```python
from build123d import *

# Parameters (mm, degrees)
SKETCH1_W                      = 60
SKETCH1_H                      = 397.5
BASE_FLANGE1_DEPTH             = 4
EDGE_FLANGE1_STRIP_W           = 18
EDGE_FLANGE1_STRIP_H           = 4
EDGE_FLANGE1_STRIP_CUT_DEPTH   = 397.5
EDGE_FLANGE1_DEPTH             = 397.5
EDGE_FLANGE2_STRIP_W           = 18
EDGE_FLANGE2_STRIP_H           = 4
EDGE_FLANGE2_STRIP_CUT_DEPTH   = 55
EDGE_FLANGE2_STRIP_2_W         = 18
EDGE_FLANGE2_STRIP_2_H         = 4
EDGE_FLANGE2_STRIP_CUT_2_DEPTH = 55
EDGE_FLANGE2_STRIP_3_W         = 18
EDGE_FLANGE2_STRIP_3_H         = 4
EDGE_FLANGE2_STRIP_CUT_3_DEPTH = 55
EDGE_FLANGE2_STRIP_4_W         = 18
EDGE_FLANGE2_STRIP_4_H         = 4
EDGE_FLANGE2_STRIP_CUT_4_DEPTH = 55
EDGE_FLANGE2_DEPTH             = 55
EDGE_FLANGE2_BEND_DEPTH        = 55
EDGE_FLANGE2_BEND_2_DEPTH      = 55
EDGE_FLANGE2_BEND_3_DEPTH      = 55
SKETCH18_R                     = 4.6
EXTRUDE1_DEPTH                 = 408.38464625
SKETCH19_R                     = 4.6
EXTRUDE2_DEPTH                 = 4
SKETCH20_R                     = 4.6
EXTRUDE3_DEPTH                 = 4


# Sheet-metal steps are written as plain solids
with BuildPart() as part:
    # Sketch1 → Base-Flange1 (new body)
    with BuildSketch(Plane(origin=(0, 0, 0), x_dir=(1, 0, 0), z_dir=(0, 1, 0))):
        Rectangle(SKETCH1_W, SKETCH1_H)
    extrude(amount=BASE_FLANGE1_DEPTH)

    # Edge-Flange1 strip (across the edge) → Edge-Flange1 strip cut (cut)
    with BuildSketch(Plane(origin=(-30, 4, -198.75), x_dir=(1, 0, 0), z_dir=(0, 0, 1))):
        with Locations((-4, -2)):
            Rectangle(EDGE_FLANGE1_STRIP_W, EDGE_FLANGE1_STRIP_H)
    extrude(amount=EDGE_FLANGE1_STRIP_CUT_DEPTH, mode=Mode.SUBTRACT)

    # Edge-Flange1 section (across the edge) → Edge-Flange1 (add)
    with BuildSketch(Plane(origin=(-30, 4, -198.75), x_dir=(1, 0, 0), z_dir=(0, 0, 1))):
        with BuildLine():
            Line((0, 1), (0, 56))
            Line((0, 56), (4, 56))
            Line((4, 56), (4, 1))
            ThreePointArc((4, 1), (4.292893219, 0.292893219), (5, 0))
            Line((5, 0), (5, -4))
            ThreePointArc((5, -4), (1.464466094, -2.535533906), (0, 1))
        make_face()
    extrude(amount=EDGE_FLANGE1_DEPTH)

    # Edge-Flange2 strip (across the edge) → Edge-Flange2 strip cut (cut)
    with BuildSketch(Plane(origin=(-30, 5, 198.75), x_dir=(0, 0, -1), z_dir=(0, 1, 0))):
        with Locations((-4, -2)):
            Rectangle(EDGE_FLANGE2_STRIP_W, EDGE_FLANGE2_STRIP_H)
    extrude(amount=EDGE_FLANGE2_STRIP_CUT_DEPTH, mode=Mode.SUBTRACT)

    # Edge-Flange2 strip 2 (across the edge) → Edge-Flange2 strip cut 2 (cut)
    with BuildSketch(Plane(origin=(30, 0, 198.75), x_dir=(0, 0, -1), z_dir=(-1, 0, 0))):
        with Locations((-4, -2)):
            Rectangle(EDGE_FLANGE2_STRIP_2_W, EDGE_FLANGE2_STRIP_2_H)
    extrude(amount=EDGE_FLANGE2_STRIP_CUT_2_DEPTH, mode=Mode.SUBTRACT)

    # Edge-Flange2 strip 3 (across the edge) → Edge-Flange2 strip cut 3 (cut)
    with BuildSketch(Plane(origin=(-30, 60, -198.75), x_dir=(0, 0, 1), z_dir=(0, -1, 0))):
        with Locations((-4, -2)):
            Rectangle(EDGE_FLANGE2_STRIP_3_W, EDGE_FLANGE2_STRIP_3_H)
    extrude(amount=EDGE_FLANGE2_STRIP_CUT_3_DEPTH, mode=Mode.SUBTRACT)

    # Edge-Flange2 strip 4 (across the edge) → Edge-Flange2 strip cut 4 (cut)
    with BuildSketch(Plane(origin=(-25, 0, -198.75), x_dir=(0, 0, 1), z_dir=(1, 0, 0))):
        with Locations((-4, -2)):
            Rectangle(EDGE_FLANGE2_STRIP_4_W, EDGE_FLANGE2_STRIP_4_H)
    extrude(amount=EDGE_FLANGE2_STRIP_CUT_4_DEPTH, mode=Mode.SUBTRACT)

    # Edge-Flange2 section (across the edge) → Edge-Flange2 (add)
    with BuildSketch(Plane(origin=(-30, 5, 198.75), x_dir=(0, 0, -1), z_dir=(0, 1, 0))):
        with BuildLine():
            Line((0, 1), (0, 36))
            Line((0, 36), (4, 36))
            Line((4, 36), (4, 1))
            ThreePointArc((4, 1), (4.292893219, 0.292893219), (5, 0))
            Line((5, 0), (5, -4))
            ThreePointArc((5, -4), (1.464466094, -2.535533906), (0, 1))
        make_face()
    extrude(amount=EDGE_FLANGE2_DEPTH)

    # Edge-Flange2 section 2 (across the edge) → Edge-Flange2 bend (add)
    with BuildSketch(Plane(origin=(30, 0, 198.75), x_dir=(0, 0, -1), z_dir=(-1, 0, 0))):
        with BuildLine():
            Line((0, 1), (0, 36))
            Line((0, 36), (4, 36))
            Line((4, 36), (4, 1))
            ThreePointArc((4, 1), (4.292893219, 0.292893219), (5, 0))
            Line((5, 0), (5, -4))
            ThreePointArc((5, -4), (1.464466094, -2.535533906), (0, 1))
        make_face()
    extrude(amount=EDGE_FLANGE2_BEND_DEPTH)

    # Edge-Flange2 section 3 (across the edge) → Edge-Flange2 bend 2 (add)
    with BuildSketch(Plane(origin=(-30, 60, -198.75), x_dir=(0, 0, 1), z_dir=(0, -1, 0))):
        with BuildLine():
            Line((0, 1), (0, 36))
            Line((0, 36), (4, 36))
            Line((4, 36), (4, 1))
            ThreePointArc((4, 1), (4.292893219, 0.292893219), (5, 0))
            Line((5, 0), (5, -4))
            ThreePointArc((5, -4), (1.464466094, -2.535533906), (0, 1))
        make_face()
    extrude(amount=EDGE_FLANGE2_BEND_2_DEPTH)

    # Edge-Flange2 section 4 (across the edge) → Edge-Flange2 bend 3 (add)
    with BuildSketch(Plane(origin=(-25, 0, -198.75), x_dir=(0, 0, 1), z_dir=(1, 0, 0))):
        with BuildLine():
            Line((0, 1), (0, 36))
            Line((0, 36), (4, 36))
            Line((4, 36), (4, 1))
            ThreePointArc((4, 1), (4.292893219, 0.292893219), (5, 0))
            Line((5, 0), (5, -4))
            ThreePointArc((5, -4), (1.464466094, -2.535533906), (0, 1))
        make_face()
    extrude(amount=EDGE_FLANGE2_BEND_3_DEPTH)

    # Sketch18 → Extrude1 (cut, through all)
    with BuildSketch(Plane.XY.offset(198.75)):
        with Locations((-46, 47.5)):
            Circle(SKETCH18_R)
        with Locations((-46, 17.5)):
            Circle(SKETCH18_R)
        with Locations((-12.5, -16)):
            Circle(SKETCH18_R)
        with Locations((17.5, -16)):
            Circle(SKETCH18_R)
    extrude(amount=-EXTRUDE1_DEPTH, mode=Mode.SUBTRACT)

    # Sketch19 → Extrude2 (cut)
    with BuildSketch(Plane(origin=(-26, 0, 0), x_dir=(0, 0, -1), z_dir=(1, 0, 0))):
        with Locations(Location((-118.75, 35, 0), (0, 0, 90))):
            Circle(SKETCH19_R)
        with Locations(Location((118.75, 35, 0), (0, 0, 90))):
            Circle(SKETCH19_R)
    extrude(amount=-EXTRUDE2_DEPTH, mode=Mode.SUBTRACT)

    # Sketch20 → Extrude3 (cut)
    with BuildSketch(Plane(origin=(0, 4, 0), x_dir=(1, 0, 0), z_dir=(0, 1, 0))):
        with Locations(Location((5, 118.75, 0), (0, 0, 270))):
            Circle(SKETCH20_R)
        with Locations(Location((5, -118.75, 0), (0, 0, 270))):
            Circle(SKETCH20_R)
    extrude(amount=-EXTRUDE3_DEPTH, mode=Mode.SUBTRACT)


solid = part.part
```
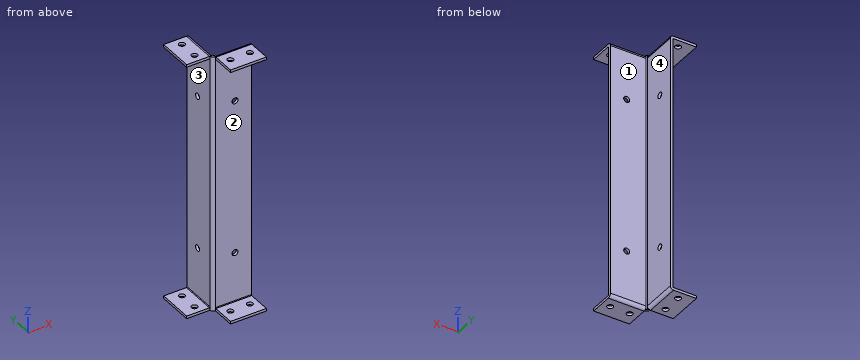
Build history of the part. All positions in model axes, mm. Face numbers are marked on the shaded views. A direction names the side the tool comes from. Give positions to 0.01 mm unless a question says otherwise; leave off trailing zeros. Loops run counter-clockwise (first coordinate to the right, second up) from the corner with the lowest first, then second, coordinate; pieces in that order, holes last. Notation, with made-up numbers: (-7.75, -7) - (47.25, -7) arc R33 ccw to (47.25, 29) - close; hole circle Ø11 at (11, 60.5). An arc over 180 degrees is marked (long way). Use a Markdown table: item, result.
(1) Which spindle directions (+Z, -Z, +X, -X, +Y, -Y) get a long thin tool onto all of the face, cutting with end or side? Do the marked faces 1 and 2. Say none if no direction does.
Taken from the geometry:
| item | result |
|---|---|
| face 1 | +Z, -Z, +X, +Y |
| face 2 | +X, -X, -Y |
(2) Pull direction Z, two halves, no side cores. Call the marked faces 3 and 4: +Z half, -Z half, draft (parallel to the pull), parting line (faces both ways), or undercut.
Taken from the geometry:
| item | result |
|---|---|
| face 3 | undercut |
| face 4 | draft |
(3) Drop flat-ended pins along their axis: pin 1 Ø10.5 at (x, y) = (-46, 17.5) entering from +Z; pin 2 Ø8.5 at (x, y) = (-46, 17.5) entering from +Z; pin 3 Ø4 at (y, z) = (-24.5, 196.5) entering from -X; pin 4 Ø10.5 at (x, z) = (5, 118.75) entering from -Y. Give the stop position or say it passes through.
Taken from the geometry:
| item | result |
|---|---|
| pin 1 | z = 198.75 |
| pin 2 | through |
| pin 3 | x = -25 |
| pin 4 | y = 0 |
(4) Wall check: line 1 along Y through (x, z) = (-46, -197); line 2 along Z through (x, y) = (-39.5, 21); line 3 along Y through (x, z) = (1, -39). Give the ranges that are in metal, low to high.
Taken from the geometry:
| item | result |
|---|---|
| line 1 | 5 to 12.9, 22.1 to 42.9, 52.1 to 60 |
| line 2 | -198.75 to -194.75, 194.75 to 198.75 |
| line 3 | 0 to 4 |
(5) Band-saw the part on C-C (x = -46). Give the cut face in (y, z), and give its area (3 significant figures).
Taken from the geometry:
| item | result |
|---|---|
| outline | (5, -198.75) - (12.9, -198.75) - (12.9, -194.75) - (5, -194.75) - close; (5, 194.75) - (12.9, 194.75) - (12.9, 198.75) - (5, 198.75) - close; (22.1, -198.75) - (42.9, -198.75) - (42.9, -194.75) - (22.1, -194.75) - close; (22.1, 194.75) - (42.9, 194.75) - (42.9, 198.75) - (22.1, 198.75) - close; (52.1, -198.75) - (60, -198.75) - (60, -194.75) - (52.1, -194.75) - close; (52.1, 194.75) - (60, 194.75) - (60, 198.75) - (52.1, 198.75) - close |
| area | 293 mm2 |
(6) Band-saw the part on D-D (x = 5). Give the cut face in (y, z).
Taken from the geometry:
| item | result |
|---|---|
| outline | (-36, -198.75) - (-1, -198.75) arc R5 ccw to (4, -193.75) - (4, -123.35) - (0, -123.35) - (0, -193.75) arc R1 cw to (-1, -194.75) - (-36, -194.75) - close; (-36, 194.75) - (-1, 194.75) arc R1 cw to (0, 193.75) - (0, 123.35) - (4, 123.35) - (4, 193.75) arc R5 ccw to (-1, 198.75) - (-36, 198.75) - close; (0, -114.15) - (4, -114.15) - (4, 114.15) - (0, 114.15) - close |
(7) Band-saw the part on B-B (y = 17.5). Give the cut face in (x, z).
Taken from the geometry:
| item | result |
|---|---|
| outline | (-66, -198.75) - (-50.6, -198.75) - (-50.6, -194.75) - (-66, -194.75) - close; (-66, 194.75) - (-50.6, 194.75) - (-50.6, 198.75) - (-66, 198.75) - close; (-41.4, -198.75) - (-31, -198.75) arc R5 ccw to (-26, -193.75) - (-26, 193.75) arc R5 ccw to (-31, 198.75) - (-41.4, 198.75) - (-41.4, 194.75) - (-31, 194.75) arc R1 cw to (-30, 193.75) - (-30, -193.75) arc R1 cw to (-31, -194.75) - (-41.4, -194.75) - close |
(8) Band-saw the part on A-A (z = -118.75). Give the cut face in (x, y).
Taken from the geometry:
| item | result |
|---|---|
| outline | (-30, 5) arc R5 ccw to (-25, 0) - (0.4, 0) - (0.4, 4) - (-25, 4) arc R1 cw to (-26, 5) - (-26, 30.4) - (-30, 30.4) - close; (-30, 39.6) - (-26, 39.6) - (-26, 60) - (-30, 60) - close; (9.6, 0) - (30, 0) - (30, 4) - (9.6, 4) - close |
